Verification items for the finished model (mm, model axes). Face numbers are marked on the shaded views. A direction names the side the tool comes from. Coordinates: 2 decimals unless noted, no trailing zeros. Order: outer loops, then holes, each group sorted by start corner. A loop starts at its lowest first (then second) coordinate and runs counter-clockwise, first axis right, second up.
Q1. Cross-section at C-C, the plane x = 17. Record the boundary of the cut face in (y, z) (3 decimals), and give its area (3 significant figures).
Q2. Set-up check for the marked faces 4 and 5: record each of +Z, -Z, +X, -X, +Y, -Y from which the full face is reachable in a straight line by a thin tool's end or side.
Q3. Depth check by flat-ended pin: P1, Ø1, axis at x = 10, z = 6.5, coming from the -Y side (3 decimals). Enter the tip coordinate at first touch or a pass-through.
Q4. Cross-section at B-B, the plane z = 14.75. Record the boundary of the cut face in (x, y) (3 decimals).
Q5. Thickness scan on line 1 (X direction, y = 8.5, z = 3.75) (3 decimals); line 2 (Y direction, x = 24.15, z = 10) (3 decimals); line 3 (Y direction, x = 9.25, z = 10.5) (3 decimals). Record the ranges inside material, lowest first.
Q6. Cross-section at D-D, the plane z = 4. Record the boundary of the cut face in (x, y) (3 decimals).
Q7. Draft check along Z on the marked faces 1, 2 and 3. Enter one of: pulls with the +Z half, pulls with the -Z half, needs draft (parallel to the pull), parting line crosses it, or undercut.
Q8. Cross-section at A-A, the plane y = 17.25. Record the boundary of the cut face in (x, z) (3 decimals).
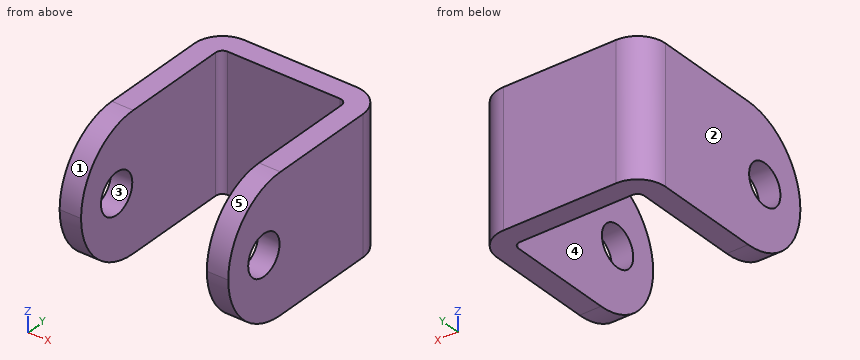
from build123d import *

# Parameters (mm, degrees)
BASE_FLANGE1_DEPTH = 20
SKETCH6_R          = 3
CUT_EXTRUDE1_DEPTH = 44.874821937
FILLET1_R          = 10


# Read off the part's stored shape, not the designer's step: Base-Flange1
with BuildPart() as part:
    # Base-Flange1 outline → Base-Flange1 (new body)
    with BuildSketch(Plane.XY):
        with BuildLine():
            Line((21.825, 25.825), (21.825, 0))
            Line((21.825, 0), (25, 0))
            Line((25, 0), (25, 25.825))
            ThreePointArc((25, 25.825), (23.777170811, 28.777170811), (20.825, 30))
            Line((20.825, 30), (4.175, 30))
            ThreePointArc((4.175, 30), (1.222829189, 28.777170811), (0, 25.825))
            Line((0, 25.825), (0, 0))
            Line((0, 0), (3.175, 0))
            Line((3.175, 0), (3.175, 25.825))
            ThreePointArc((3.175, 25.825), (3.467893219, 26.532106781), (4.175, 26.825))
            Line((4.175, 26.825), (20.825, 26.825))
            ThreePointArc((20.825, 26.825), (21.532106781, 26.532106781), (21.825, 25.825))
        make_face()
    extrude(amount=BASE_FLANGE1_DEPTH)

    # Sketch6 → Cut-Extrude1 (cut, through all)
    with BuildSketch(Plane.ZY):
        with Locations((10, 6.825)):
            Circle(SKETCH6_R)
    extrude(amount=-CUT_EXTRUDE1_DEPTH, mode=Mode.SUBTRACT)

    # Fillet1
    fillet1_edges = [part.edges().sort_by_distance(p)[0] for p in [
        (23.4125, 0, 20),
        (23.4125, 0, 0),
        (1.5875, 0, 0),
        (1.5875, 0, 20),
    ]]
    fillet(fillet1_edges, radius=FILLET1_R - 0.0001)  # a hair under: the kernel refuses the full size


solid = part.part
Check values:
1. outline: (26.825, 0) - (30, 0) - (30, 20) - (26.825, 20) - close
1. area: 63.5 mm2
2. face 4: +Z, -Z, -Y
2. face 5: +Z, +X, -X, -Y
3. P1: stops at y = 26.825
4. outline: (0, 1.2) - (3.175, 1.2) - (3.175, 25.825) arc R1 cw to (4.175, 26.825) - (20.825, 26.825) arc R1 cw to (21.825, 25.825) - (21.825, 1.2) - (25, 1.2) - (25, 25.825) arc R4.175 ccw to (20.825, 30) - (4.175, 30) arc R4.175 ccw to (0, 25.825) - close
5. line 1: x = 0 to 3.175, 21.825 to 25
5. line 2: y = 0 to 3.825, 9.825 to 28.35
5. line 3: y = 26.825 to 30
6. outline: (0, 2) - (3.175, 2) - (3.175, 25.825) arc R1 cw to (4.175, 26.825) - (20.825, 26.825) arc R1 cw to (21.825, 25.825) - (21.825, 2) - (25, 2) - (25, 25.825) arc R4.175 ccw to (20.825, 30) - (4.175, 30) arc R4.175 ccw to (0, 25.825) - close
7. face 1: pulls with the +Z half
7. face 2: needs draft
7. face 3: undercut
8. outline: (0, 0) - (3.175, 0) - (3.175, 20) - (0, 20) - close; (21.825, 0) - (25, 0) - (25, 20) - (21.825, 20) - close
